Verification items for the finished model (mm, model axes). A direction names the side the tool comes from. Round coordinates to 2 decimals unless told otherwise and drop trailing zeros. Write each loop counter-clockwise with the first axis right and the second up, starting at its lowest first coordinate (ties: lowest second). Pieces come first, ordered by that corner, then holes.
Autodesk Inventor part; units mm, degrees
ref_plane "YZ Plane" through (0, 0, 0) normal (1, 0, 0) x (0, 1, 0)
ref_plane "XZ Plane" through (0, 0, 0) normal (0, 1, 0) x (-1, 0, 0)
ref_plane "XY Plane" through (0, 0, 0) normal (0, 0, 1) x (1, 0, 0)
sketch "Sketch1" plane through (0, 0, 0) normal (0, 1, 0) x (-1, 0, 0)
  line L0 (85, -50) -> (65, -50)
  line L1 (-85, -50) -> (-85, 0)
  line L2 (-85, 0) -> (85, 0)
  line L3 (85, 0) -> (85, -50)
  line L4 (85, -50) -> (-85, 0) construction
  line L5 (-85, -50) -> (85, 0) construction
  arc A0 (65, -50) -> (-65, -50) centre (0, -126.0208) ccw
  line L6 (65, -50) -> (-65, -50) construction
  line L7 (-65, -50) -> (-85, -50)
  line L8 (65, -28.5948) -> (65, -14)
  line L9 (63, -12) -> (30.2021, -12)
  arc A1 (61.914, -30.2742) -> (29.6815, -15.931) centre (0, -126.0208) ccw
  line L10 (0, 0) -> (0, -25)
  arc A2 (30.2021, -12) -> (29.6815, -15.931) centre (30.2021, -14) ccw
  arc A3 (65, -14) -> (63, -12) centre (63, -14) ccw
  arc A4 (61.914, -30.2742) -> (65, -28.5948) centre (63, -28.5948) ccw
  line L11 (-65, -28.5948) -> (-65, -14)
  line L12 (-63, -12) -> (-30.2021, -12)
  arc A5 (-29.6815, -15.931) -> (-61.914, -30.2742) centre (0, -126.0208) ccw
  arc A6 (-29.6815, -15.931) -> (-30.2021, -12) centre (-30.2021, -14) ccw
  arc A7 (-63, -12) -> (-65, -14) centre (-63, -14) ccw
  arc A8 (-65, -28.5948) -> (-61.914, -30.2742) centre (-63, -28.5948) ccw
  point P0 (0, -25)
  point P1 (0, -25)
  point P2 (65, -32.3419)
  point P3 (0, -12)
  dimension "d0" = 170
  dimension "d1" = 50
  dimension "d2" = 26
  dimension "d3" = 20
  dimension "d4" = 12
  dimension "d5" = 20
  dimension "d6" = 2
extrude "Extrusion1" add sketch "Sketch1" along normal mid plane 3.175
sketch "Sketch2" plane through (0, 1.5875, 0) normal (0, 1, 0) x (1, 0, 0)
  line L0 (-85, 0) -> (85, 0)
  line L1 (-85, 50) -> (-85, 0)
  line L2 (-65, 50) -> (-85, 50)
  line L3 (0, 0) -> (0, 15.0505)
  point P0 (-75, 10)
  point P1 (-75, 40)
  point P2 (75, 10)
  point P3 (75, 40)
  dimension "d9" = 10
  dimension "d10" = 10
  dimension "d11" = 10
hole "Hole1" at (-75, 1.5875, -10) at (-75, 1.5875, -40) at (75, 1.5875, -40) at (75, 1.5875, -10) direction (0, -1, 0) diameter 5 end through all
sketch "Sketch4" plane through (0, 1.5875, 0) normal (0, 1, 0) x (1, 0, 0)
  line L0 (-85, 50) -> (-85, 0)
  arc A0 (-30.2021, 12) -> (-29.6815, 15.931) centre (-30.2021, 14) ccw
  line L1 (-85, 0) -> (85, 0)
  point P0 (0, 0)
  point P1 (-5, 10)
  dimension "d29" = 80
  dimension "d37" = 10
hole "Hole3" at (-5, 1.5875, -10) direction (0, -1, 0) diameter 5.5118 depth 14.2 tip angle 118
properties part number "Upper Cross Bracket" material "Aluminum 6061"
Q1. Tool access check on faces 1 (the cylindrical face through (0.991, -0.022, -26.005)), 2 (the cylindrical face through (-46.13, -0.02, -21.75)). Record the directions out of +Z, -Z, +X, -X, +Y, -Y that give a thin tool (end or side, any length) a straight path to the whole face; none if there is none.
Recorded:
face 1: -Z, +Y, -Y
face 2: +Y, -Y
Q2. Depth check by flat-ended pin: P1, Ø7, axis at x = -5, z = -10, coming from the +Y side; P2, Ø4, axis at x = 75, z = -10, coming from the +Y side; P3, Ø1.6, axis at x = -47.5, y = 0.5, coming from the -Z side (3 decimals). Enter the tip coordinate at first touch or a pass-through.
Recorded:
P1: stops at y = 1.59
P2: passes through
P3: stops at z = -38.435
Q3. Sectioned sample at B-B (z = -10). Enter the section's corners in (x, y).
Recorded:
outline: (-85, -1.59) - (-77.5, -1.59) - (-77.5, 1.59) - (-85, 1.59) - close; (-72.5, -1.59) - (-7.76, -1.59) - (-7.76, 1.59) - (-72.5, 1.59) - close; (-2.24, -1.59) - (72.5, -1.59) - (72.5, 1.59) - (-2.24, 1.59) - close; (77.5, -1.59) - (85, -1.59) - (85, 1.59) - (77.5, 1.59) - close
Q4. Release check for a two-part mould opening along Z. For faces 3 (the flat face through (75, 0, -50)), 4 (the flat face through (47, 0, -12)), 5 (the flat face through (-85, 0, -25)) record: released by +Z, released by -Z, zero draft, split by the parting line, or undercut.
Recorded:
face 3: released by -Z
face 4: undercut
face 5: zero draft
Q5. Material ranges on line 1 along X through (y, z) = (-0.7, -10); line 2 along Z through (x, y) = (75, 0.4); line 3 along X through (y, z) = (-0.9, -40), recorded low to high.
Recorded:
line 1: x = -85 to -77.5, -72.5 to -7.76, -2.24 to 72.5, 77.5 to 85
line 2: z = -50 to -42.5, -37.5 to -12.5, -7.5 to 0
line 3: x = -85 to -77.5, -72.5 to -51.04, 51.04 to 72.5, 77.5 to 85
Q6. Sectioned sample at A-A (y = -0.95). Enter the section's corners in (x, z).
Recorded:
outline: (-85, -50) - (-65, -50) arc R100.02 cw to (65, -50) - (85, -50) - (85, 0) - (-85, 0) - close; hole circle Ø5 at (-75, -40); hole circle Ø5 at (-75, -10); hole (-65, -28.59) arc R2 ccw to (-61.91, -30.27) arc R114.02 cw to (-29.68, -15.93) arc R2 ccw to (-30.2, -12) - (-63, -12) arc R2 ccw to (-65, -14) - close; hole circle Ø5.51 at (-5, -10); hole (29.68, -15.93) arc R114.02 cw to (61.91, -30.27) arc R2 ccw to (65, -28.59) - (65, -14) arc R2 ccw to (63, -12) - (30.2, -12) arc R2 ccw to start; hole circle Ø5 at (75, -40); hole circle Ø5 at (75, -10)
Q7. Sectioned sample at C-C (x = -5). Enter the section's corners in (y, z), plus the area to 3 significant figures.
Recorded:
outline: (-1.59, -26.13) - (1.59, -26.13) - (1.59, -12.76) - (-1.59, -12.76) - close; (-1.59, -7.24) - (1.59, -7.24) - (1.59, 0) - (-1.59, 0) - close
area: 65.4 mm2
Q8. Sectioned sample at D-D (z = -21). Enter the section's corners in (x, y).
Recorded:
outline: (-85, -1.59) - (-65, -1.59) - (-65, 1.59) - (-85, 1.59) - close; (-44.4, -1.59) - (44.4, -1.59) - (44.4, 1.59) - (-44.4, 1.59) - close; (65, -1.59) - (85, -1.59) - (85, 1.59) - (65, 1.59) - close
